from build123d import *

# Parameters (mm, degrees)
CUT_EXTRUDE1_START = -3
CUT_EXTRUDE1_DEPTH = 12
CIRPATTERN1_COUNT  = 15


with BuildPart() as part:
    # Sketch1 → Revolve1 (revolve)
    with BuildSketch(Plane.XY, mode=Mode.PRIVATE) as revolve1_sk:
        with BuildLine():
            Line((-10.5, 3), (10.5, 3))
            Line((10.5, 3), (10.5, 14))
            Line((10.5, 14), (9.75, 14))
            ThreePointArc((9.75, 14), (9.191617437, 12.818070474), (9, 11.525))
            Line((9, 11.525), (-3, 11.525))
            ThreePointArc((-3, 11.525), (-3.191617437, 12.818070474), (-3.75, 14))
            Line((-3.75, 14), (-4.5, 14))
            Line((-4.5, 14), (-4.5, 8))
            Line((-4.5, 8), (-10.5, 8))
            Line((-10.5, 8), (-10.5, 3))
        make_face()
    revolve(revolve1_sk.sketch.rotate(Axis((-10.5, 0, 0), (1, 0, 0)), 90), axis=Axis((-10.5, 0, 0), (1, 0, 0)))

    # Sketch3 → Cut-Extrude1 (cut)
    with BuildSketch(Plane(origin=(0, 0, 0), x_dir=(0, 0, -1), z_dir=(1, 0, 0)).offset(CUT_EXTRUDE1_START)):
        with BuildLine():
            Line((-1.325, 11.448580698), (-0.901692109, 10.285551825))
            Line((-0.901692109, 10.285551825), (0.901692109, 10.285551825))
            Line((0.901692109, 10.285551825), (1.325, 11.448580698))
            ThreePointArc((1.325, 11.448580698), (0, 11.525), (-1.325, 11.448580698))
        make_face()
    cut_extrude1 = extrude(amount=CUT_EXTRUDE1_DEPTH, mode=Mode.SUBTRACT)

    # CirPattern1: Cut-Extrude1 ×15 about axis
    cirpattern1_axis = Axis((0, 0, 0), (1, 0, 0))
    for i in range(1, CIRPATTERN1_COUNT):
        add(cut_extrude1.rotate(cirpattern1_axis, i * 360 / CIRPATTERN1_COUNT), mode=Mode.SUBTRACT)


solid = part.part
Can you work these out from the model? Positions are in its coordinate system, mm. A direction names the side the tool comes from. Coordinates: 2 decimals unless noted, no trailing zeros. Use one line per item in the form item = value.
Q1. Which directions (+Z, -Z, +X, -X, +Y, -Y) give clear straight access to the entire face, cutting with the end or side of a thin tool? Please do faces 1 (the face through (2.92, 10.86, -1.11)), 2 (the face through (2.916, -9.438, -5.484)), 3 (the face through (-3, 3, 10)), 4 (the face through (2.916, -11.525, 0.015)).
From the geometry:
face_1 = +Y
face_2 = -Z
face_3 = +Z
face_4 = -Y
Q2. I need wall thicknesses on L1, parallel to Y at x = -0.75, z = 0 (3 decimals); L2, parallel to X at y = -3.75, z = 10; L3, parallel to X at y = -11.5, z = 6.5. Which ranges of each line are inside material? Lowest first, please.
From the geometry:
L1 = -11.525 to -3, 3 to 10.286
L2 = -4.5 to 10.5
L3 = -4.5 to -3.33, 9.33 to 10.5
Q3. Will these pins go through, and if not, where does the flat tip stop? P1, Ø0.9, axis at x = 1, z = 0, coming from the +Y side; P2, Ø1.1, axis at y = -6, z = 9, coming from the -X side; P3, Ø1.5, axis at x = 0.5, z = 7, coming from the -Y side.
From the geometry:
P1 = 10.29
P2 = -4.5
P3 = -8.45
Q4. We'd pull the mould along Y, two halves only. Please class faces 5 (the face through (2.916, -2.239, -10.683)), 6 (the face through (2.916, -10.391, 3.344)), 7 (the face through (9, -11, 2)), 8 (the face through (-7.54, 7.81, -1.73)): released by +Y, released by -Y, zero draft, split by the parting line, or undercut.
From the geometry:
face_5 = undercut
face_6 = released by -Y
face_7 = zero draft
face_8 = split by the parting line
